Could you check a few things on this model? Use its own coordinates, in mm. A direction names the side the tool comes from. Round coordinates to 2 decimals unless told otherwise and drop trailing zeros. Write each loop counter-clockwise with the first axis right and the second up, starting at its lowest first coordinate (ties: lowest second). Pieces come first, ordered by that corner, then holes. Notation, with made-up numbers: (17, 20) -> (47, 20) arc R9 cw to (47, 24) -> close; hole circle Ø10 at (78, -40). An arc over 180 degrees is marked (long way). Return JSON: item names as keys, results as strings.
from build123d import *

# Parameters (mm, degrees)
F1_DEPTH = 63.5
F2_DEPTH = 25.4
F3_DEPTH = 7.9375
F4_R     = 27.8728367349
F5_DEPTH = 63.5
F6_DEPTH = 42.418
F7_R     = 6.35


with BuildPart() as f1:
    # F0 (on Front) → F1 (new body, symmetric)
    with BuildSketch(Plane.XZ):
        Polygon((41.275, -10.04768112), (41.275, 10.04768112), (22.225, 10.04768112), (-41.275, 10.04768112), (-41.275, -10.04768112), align=None)
    extrude(amount=F1_DEPTH, both=True)

    # F0 (on Front) → F2 (join, symmetric)
    with BuildSketch(Plane.XZ):
        with BuildLine():
            Line((22.225, 10.04768112), (41.275, 10.04768112))
            Line((41.275, 10.04768112), (41.275, 32.7466142374))
            ThreePointArc((41.275, 32.7466142374), (44.0462635088, 40.2080273698), (51.0162711539, 44.0514087971))
            Line((51.0162711539, 44.0514087971), (62.7183187845, 44.0514087971))
            Line((62.7183187845, 44.0514087971), (62.7183187845, 63.1014087971))
            Line((62.7183187845, 63.1014087971), (49.9424132783, 63.1014087971))
            add(Edge.make_bspline(
                [(35.3324258873, 57.7911980863), (40.4505273994, 60.0549715303), (45.3379731216, 61.8597652076), (49.9424132783, 63.1014087971)],
                knots=[0.5056708744, 0.5056708744, 0.5056708744, 0.5056708744, 0.620438237, 0.620438237, 0.620438237, 0.620438237], degree=3))
            ThreePointArc((35.3324258873, 57.7911980863), (25.6999386791, 46.8802248302), (22.225, 32.7466142374))
            Line((22.225, 32.7466142374), (22.225, 10.04768112))
        make_face()
    extrude(amount=F2_DEPTH, both=True)

    # F0 (on Front) → F3 (join, symmetric)
    with BuildSketch(Plane.XZ):
        with BuildLine():
            Line((-41.275, 10.04768112), (22.225, 10.04768112))
            Line((22.225, 10.04768112), (22.225, 32.7466142374))
            ThreePointArc((22.225, 32.7466142374), (25.6999386791, 46.8802248302), (35.3324258873, 57.7911980863))
            add(Edge.make_bspline(
                [(-41.275, 10.04768112), (-14.2465956817, 28.9322887665), (12.7818086366, 47.816896413), (35.3324258873, 57.7911980863)],
                knots=[0, 0, 0, 0, 0.5056708744, 0.5056708744, 0.5056708744, 0.5056708744], degree=3))
        make_face()
    extrude(amount=F3_DEPTH, both=True)

    # F4 (on Top) → F5 (join)
    with BuildSketch(Plane.XY):
        with Locations((74.4178891182, 0)):
            Circle(F4_R)
    extrude(amount=F5_DEPTH)

    # F6 (cut): a face of the model
    f6_faces = [f1.faces().sort_by_distance(p)[0] for p in [
        (74.4178891182, 0, 0),
    ]]
    extrude(f6_faces, amount=-F6_DEPTH, mode=Mode.SUBTRACT)

    # F7
    f7_edges = [f1.edges().sort_by_distance(p)[0] for p in [
        (-41.275, -63.5, 0),
        (-41.275, 63.5, 0),
        (41.275, -63.5, 0),
        (41.275, 63.5, 0),
    ]]
    fillet(f7_edges, radius=F7_R)


solid = f1.part
1) Thinking about a two-plate mould opening in X: for faces 5 (the face through (39.464, 61.59, 0.141)), 6 (the face through (54, -23, 44.051)), 7 (the face through (-39.365, -61.689, -0.141)), 8 (the face through (54, -22, 63.101)), which applies, pulls with the +X half, pulls with the -X half, needs draft (parallel to the pull), parting line crosses it, or undercut?
Return value:
{"face 5": "pulls with the +X half", "face 6": "undercut", "face 7": "pulls with the -X half", "face 8": "needs draft"}
2) I want a section at B-B, the plane y = -42.5. Please give me the cut outline in (x, z) (3 decimals), and give its area (3 significant figures).
Return value:
{"outline": "(-41.275, -10.048) -> (41.275, -10.048) -> (41.275, 10.048) -> (-41.275, 10.048) -> close", "area": "1,660 mm²"}
3) If I drill on probe 1 along Z at (x, y) = (15, -35); probe 2 along Z at (x, y) = (59, -15); probe 3 along Y at (x, z) = (4.5, 11.5), over which ranges is the centre line in solid material (lowest first)? Write a range as [from, to].
Return value:
{"probe 1": "[-10.05, 10.05]", "probe 2": "[42.42, 63.5]", "probe 3": "[-7.94, 7.94]"}
4) Will these pins go through, and if not, where does the flat tip stop? pin 1 Ø8 at (x, y) = (56.5, 21.5) entering from -Z; pin 2 Ø5 at (y, z) = (-21, 29.5) entering from +X (3 decimals); pin 3 Ø5 at (y, z) = (20, 17.5) entering from -X (3 decimals); pin 4 Ø12 at (x, z) = (50.5, 33) entering from -Y.
Return value:
{"pin 1": "z = 42.42", "pin 2": "x = 41.275", "pin 3": "x = 22.225", "pin 4": "through"}
5) For faces 1 (the face through (0, -63.5, 0)), 2 (the face through (54, 22, 63.101)), 3 (the face through (74, 0, 42.418)), 4 (the face through (38, -25.4, 43)), which set-ups out of +Z, -Z, +X, -X, +Y, -Y let a thin tool reach every point of the face, with its end or its side?
Return value:
{"face 1": "+Z, -Z, +X, -X, -Y", "face 2": "+Z, -X, +Y", "face 3": "-Z, +X, +Y, -Y", "face 4": "+Z, -X, -Y"}
6) I want a section at A-A, the plane z = 1.5. Please give me the cut outline in (x, y) (3 decimals), and give its area (3 significant figures).
Return value:
{"outline": "(-41.275, -57.15) arc R6.35 ccw to (-34.925, -63.5) -> (34.925, -63.5) arc R6.35 ccw to (41.275, -57.15) -> (41.275, 57.15) arc R6.35 ccw to (34.925, 63.5) -> (-34.925, 63.5) arc R6.35 ccw to (-41.275, 57.15) -> close", "area": "10,400 mm²"}
